from build123d import *

# Parameters (mm, degrees)
BOSS_EXTRUDE1_DEPTH = 16
SKETCH4_R           = 6
CUT_EXTRUDE1_DEPTH  = 7
SKETCH5_R           = 3.2
CUT_EXTRUDE2_DEPTH  = 11
FILLET1_R           = 0.4


with BuildPart() as part:
    # Sketch3 → Boss-Extrude1 (new body)
    with BuildSketch(Plane.XY):
        Polygon((0, 0), (0, -32), (25, -32), (32.331439149, -22.5), (32.331439149, -9.5), (25, 0), align=None)
    extrude(amount=BOSS_EXTRUDE1_DEPTH)

    # Sketch4 → Cut-Extrude1 (cut)
    with BuildSketch(Plane.XY.offset(16)):
        with Locations((16.165719575, -16)):
            Circle(SKETCH4_R)
    extrude(amount=-CUT_EXTRUDE1_DEPTH, mode=Mode.SUBTRACT)

    # Sketch5 → Cut-Extrude2 (cut)
    with BuildSketch(Plane.XY.offset(9)):
        with Locations((16.165719575, -16)):
            Circle(SKETCH5_R)
    extrude(amount=-CUT_EXTRUDE2_DEPTH, mode=Mode.SUBTRACT)

    # Fillet1
    fillet1_edges = [part.edges().sort_by_distance(p)[0] for p in [
        (25, 0, 8),
        (32.331439149, -9.5, 8),
        (32.331439149, -22.5, 8),
        (25, -32, 8),
        (0, -32, 8),
        (0, 0, 8),
        (12.5, -32, 16),
        (28.665719575, -27.25, 16),
        (10.165719575, -16, 9),
        (10.165719575, -16, 16),
        (32.331439149, -16, 16),
        (28.665719575, -4.75, 16),
        (12.965719575, -16, 0),
        (12.965719575, -16, 9),
        (12.5, 0, 16),
        (28.665719575, -4.75, 0),
        (32.331439149, -16, 0),
        (28.665719575, -27.25, 0),
        (12.5, -32, 0),
        (0, -16, 0),
        (12.5, 0, 0),
        (0, -16, 16),
    ]]
    fillet(fillet1_edges, radius=FILLET1_R)


solid = part.part
Check sheet for the modelled part. Datum: model origin and axes. Units: mm. A direction names the side the tool comes from. Round coordinates to 2 decimals unless told otherwise and drop trailing zeros. Order: outer loops, then holes, each group sorted by start corner. A loop starts at its lowest first (then second) coordinate and runs counter-clockwise, first axis right, second up.
Q1. Scan lines: L1, parallel to X at y = -16.5, z = 10.5; L2, parallel to X at y = -14, z = 11.5; L3, parallel to Z at x = 11.5, y = -18. Record each from-to range of solid material in increasing order.
Filled sheet:
L1: x = 0 to 10.19, 22.14 to 32.33
L2: x = 0 to 10.51, 21.82 to 32.33
L3: z = 0 to 9
Q2. Cross-section at B-B, the plane z = 5. Enter the section's corners in (x, y), plus the area to 3 significant figures.
Filled sheet:
outline: (0, -31.6) arc R0.4 ccw to (0.4, -32) - (24.8, -32) arc R0.4 ccw to (25.12, -31.84) - (32.25, -22.61) arc R0.4 ccw to (32.33, -22.36) - (32.33, -9.64) arc R0.4 ccw to (32.25, -9.39) - (25.12, -0.16) arc R0.4 ccw to (24.8, 0) - (0.4, 0) arc R0.4 ccw to (0, -0.4) - close; hole circle Ø6.4 at (16.17, -16)
area: 933 mm2
Q3. Cross-section at A-A, the plane y = -16. Enter the section's corners in (x, z), plus the area to 3 significant figures.
Filled sheet:
outline: (0, 0.4) arc R0.4 ccw to (0.4, 0) - (12.57, 0) arc R0.4 ccw to (12.97, 0.4) - (12.97, 8.6) arc R0.4 ccw to (12.57, 9) - (10.57, 9) arc R0.4 cw to (10.17, 9.4) - (10.17, 15.6) arc R0.4 ccw to (9.77, 16) - (0.4, 16) arc R0.4 ccw to (0, 15.6) - close; (19.37, 0.4) arc R0.4 ccw to (19.77, 0) - (31.93, 0) arc R0.4 ccw to (32.33, 0.4) - (32.33, 15.6) arc R0.4 ccw to (31.93, 16) - (22.57, 16) arc R0.4 ccw to (22.17, 15.6) - (22.17, 9.4) arc R0.4 cw to (21.77, 9) - (19.77, 9) arc R0.4 ccw to (19.37, 8.6) - close
area: 375 mm2
Q4. Depth check by flat-ended pin: P1, Ø6, axis at x = 16.17, y = -16, coming from the +Z side. Enter the tip coordinate at first touch or a pass-through.
Filled sheet:
P1: passes through
Q5. Set-up check for faces 4 (the face through (11.743, -11.945, 12.543)), 5 (the face through (12, -16, 0)): record each of +Z, -Z, +X, -X, +Y, -Y from which the full face is reachable in a straight line by a thin tool's end or side.
Filled sheet:
face 4: +Z
face 5: -Z, +X, -X, +Y, -Y
Q6. Draft check along X on faces 1 (the face through (28.734, -4.838, 7.894)), 2 (the face through (20, -16, 9)), 3 (the face through (13, 0, 8)). Enter one of: pulls with the +X half, pulls with the -X half, needs draft (parallel to the pull), parting line crosses it, or undercut.
Filled sheet:
face 1: pulls with the +X half
face 2: undercut
face 3: needs draft
